Verification items for the finished model (mm, model axes). A direction names the side the tool comes from. Coordinates: 2 decimals unless noted, no trailing zeros. Loops run counter-clockwise (first coordinate to the right, second up) from the corner with the lowest first, then second, coordinate; pieces in that order, holes last. Notation, with made-up numbers: (-13.5, -6) -> (-8.5, -6) arc R23 cw to (-8.5, 17) -> close; hole circle Ø10 at (-29, 66.25). An arc over 180 degrees is marked (long way). Write item = value, one per line.
```python
from build123d import *

# Parameters (mm, degrees)
EXTRUDE012_DEPTH = 10
EXTRUDE011_DEPTH = 40


with BuildPart() as extrude012:
    # Sketch006 → Extrude012 (new body)
    with BuildSketch(Plane.XY):
        with BuildLine():
            ThreePointArc((2, 57), (0.585786, 56.414214), (0, 55))
            Line((0, 55), (0, 0))
            Line((0, 0), (20, 0))
            Line((20, 0), (20, 55))
            ThreePointArc((20, 55), (19.414214, 56.414214), (18, 57))
            Line((2, 57), (18, 57))
        make_face()
    extrude(amount=EXTRUDE012_DEPTH)


with BuildPart() as body002:
    # Sketch007 → Extrude011 (new body)
    with BuildSketch(Plane.YZ):
        with BuildLine():
            Line((0, 0), (57, 0))
            Line((57, 0), (57, 0.4))
            Line((57, 0.4), (52, 0.4))
            ThreePointArc((47, 1.5), (49.440215, 0.678249), (52, 0.4))
            Line((47, 1.5), (0, 1.5))
            Line((0, 1.5), (0, 0))
        make_face()
    extrude(amount=EXTRUDE011_DEPTH)

    # Common: intersect Extrude012
    add(extrude012.part, mode=Mode.INTERSECT)


solid = body002.part
```
1) Sectioned sample at B-B, the plane y = 53. Record the cut outline in (x, z), plus the area to 3 significant figures.
Ans:
outline = (0, 0) -> (20, 0) -> (20, 0.4) -> (0, 0.4) -> close
area = 8.00 mm2
2) Depth check by flat-ended pin: pin 1 Ø5.5 at (x, y) = (8.5, 55.5) entering from +Z. Enter the tip coordinate at first touch or a pass-through.
Ans:
pin_1 = 0.4
3) Sectioned sample at C-C, the plane z = 0.75. Record the cut outline in (x, y).
Ans:
outline = (0, 0) -> (20, 0) -> (20, 49.13) -> (0, 49.13) -> close
4) Tool access check on faces 1 (the face through (0.6, 56.43, 0.2)), 2 (the face through (10, 55, 0.4)). Record the directions out of +Z, -Z, +X, -X, +Y, -Y that give a thin tool (end or side, any length) a straight path to the whole face; none if there is none.
Ans:
face_1 = +Z, -Z, -X, +Y
face_2 = +Z, +X, -X, +Y
5) Material ranges on line 1 (Z direction, x = 11.5, y = 54); line 2 (Y direction, x = 7.5, z = 1.35); line 3 (Z direction, x = 11.75, y = 47.5), recorded low to high.
Ans:
line_1 = 0 to 0.4
line_2 = 0 to 47.34
line_3 = 0 to 1.28
6) Sectioned sample at A-A, the plane x = 8.25. Record the cut outline in (y, z), plus the area to 3 significant figures.
Ans:
outline = (0, 0) -> (57, 0) -> (57, 0.4) -> (52, 0.4) arc R11.91 cw to (47, 1.5) -> (0, 1.5) -> close
area = 76.3 mm2
